For this review, use the dimensioned drawing (mm, ordinates from the lowest corner) and the shaded views. A direction names the side the tool comes from. Give positions to 0.01 mm unless a question says otherwise; leave off trailing zeros. Order: outer loops, then holes, each group sorted by start corner. A loop starts at its lowest first (then second) coordinate and runs counter-clockwise, first axis right, second up. Notation, with made-up numbers: (-28.5, 38) - (10.5, 38) arc R19 ccw to (10.5, 56) - close; hole circle Ø3 at (35.25, 30). An arc over 180 degrees is marked (long way). One line per item, written item: value.
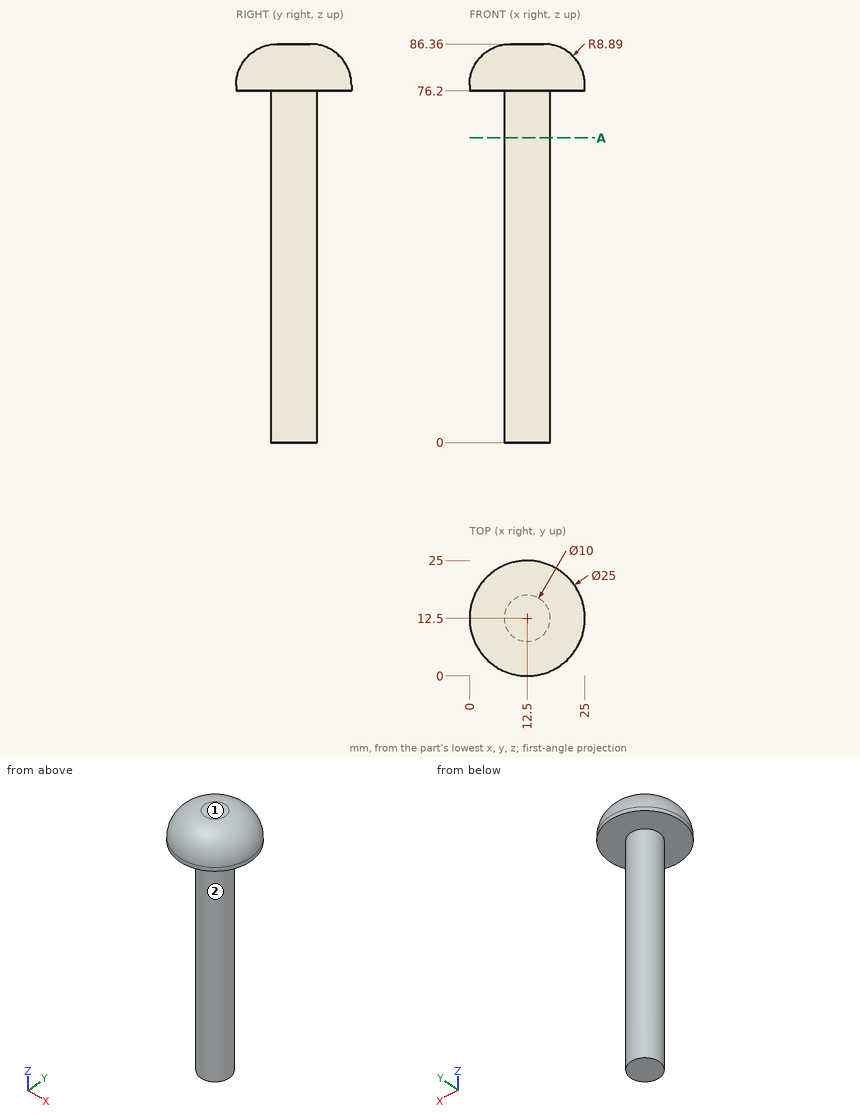
(1) Machinability: for the marked faces 1 and 2, which of the approach directions +Z, -Z, +X, -X, +Y, -Y give a long, thin tool a straight path to every point of the face, cutting with its end or side? Answer none if there is none.
Answers below:
face 1: +Z, +X, -X, +Y, -Y
face 2: -Z
(2) For P1, Ø5, axis at y = 3, z = 17.5, coming from the -X side; P2, Ø1, axis at y = 17.5, z = 72, coming from the +X side; P3, Ø8, axis at x = 14, z = 15.5, coming from the -Y side; P4, Ø12, axis at x = 21.5, y = 3, coming from the +Z side, all flat-tipped, find the tip position at first contact; note any pin that passes through.
Answers below:
P1: passes through
P2: stops at x = 14.68
P3: stops at y = 7.5
P4: stops at z = 85.65
(3) Wall thickness on line 1 (Z direction, x = 9.5, y = 15.25); line 2 (X direction, y = 11.5, z = 8.5): over which ranges is each line inside the solid? List them lowest first. Write a range as from..to.
Answers below:
line 1: z = 0..86.35
line 2: x = 7.6..17.4
(4) Take a section at A-A (z = 66). Write out the cut boundary in (x, y), then the cut area to 3 significant figures.
Answers below:
outline: circle Ø10 at (12.5, 12.5)
area: 78.5 mm^2
